Geometry: final body of the model. Coordinates: model frame, mm. A direction names the side the tool comes from. Round coordinates to 2 decimals unless told otherwise and drop trailing zeros. Loops run counter-clockwise (first coordinate to the right, second up) from the corner with the lowest first, then second, coordinate; pieces in that order, holes last. Notation, with made-up numbers: M -36.5,7 L -15.5,7 A13 cw -15.5,11 Z; hole C -12,84 d8. An arc over 180 degrees is marked long. Answer as a JSON object with one key per item and string values.
```python
from build123d import *

# Parameters (mm, degrees)
SKETCH1_R           = 2.5
BOSS_EXTRUDE1_DEPTH = 3.5
SKETCH2_R           = 1.5
CUT_EXTRUDE1_DEPTH  = 77.148499601
FILLET1_R           = 10
SKETCH5_R           = 15.25
SKETCH5_R_2         = 3
CUT_EXTRUDE4_DEPTH  = 77.148499601


with BuildPart() as part:
    # Sketch1 → Boss-Extrude1 (new body)
    with BuildSketch(Plane.XY):
        with BuildLine():
            Line((0, -19), (30, -19))
            Line((30, -19), (64.201367261, 15.201367261))
            Line((64.201367261, 15.201367261), (58.615223689, 20.787510832))
            Line((58.615223689, 20.787510832), (31.745166004, -6.082546853))
            Line((31.745166004, -6.082546853), (17.320187668, 8.342431483))
            Line((17.320187668, 8.342431483), (44.190245353, 35.212489168))
            Line((44.190245353, 35.212489168), (38.604101782, 40.798632739))
            Line((38.604101782, 40.798632739), (16.805469042, 19))
            Line((16.805469042, 19), (0, 19))
            ThreePointArc((0, 19), (-19, 0), (0, -19))
        make_face()
        Circle(SKETCH1_R, mode=Mode.SUBTRACT)
    extrude(amount=BOSS_EXTRUDE1_DEPTH)

    # Sketch2 → Cut-Extrude1 (cut, through all)
    with BuildSketch(Plane.XY.offset(3.5)):
        with Locations((38.878105659, 35.574881393)):
            Circle(SKETCH2_R)
        with Locations((58.977615915, 15.475371138)):
            Circle(SKETCH2_R)
    extrude(amount=-CUT_EXTRUDE1_DEPTH, mode=Mode.SUBTRACT)

    # Fillet1
    fillet1_edges = [part.edges().sort_by_distance(p)[0] for p in [
        (30, -19, 1.75),
        (16.805469042, 19, 1.75),
    ]]
    fillet(fillet1_edges, radius=FILLET1_R)

    # Sketch5 → Cut-Extrude4 (cut, through all)
    with BuildSketch(Plane.XY.offset(3.5)):
        Circle(SKETCH5_R)
        with Locations((38.878105659, 35.574881393)):
            Circle(SKETCH5_R_2)
        with Locations((58.977615915, 15.475371138)):
            Circle(SKETCH5_R_2)
    extrude(amount=-CUT_EXTRUDE4_DEPTH, mode=Mode.SUBTRACT)


solid = part.part
```
1) Line query: probe 1 along X at (y, z) = (-2.5, 2.85); probe 2 along X at (y, z) = (1.5, 1.55); probe 3 along X at (y, z) = (-7, 0.8). Output: solid intervals per line, ascending.
Geometry results:
{"probe 1": "-18.83 to -15.04, 15.04 to 28.16, 35.33 to 46.5", "probe 2": "-18.94 to -15.18, 15.18 to 24.16, 39.33 to 50.5", "probe 3": "-17.66 to -13.55, 13.55 to 42"}
2) Pull-direction query (X, two-part tool) for faces 1 (the face through (22, 2, 0)), 2 (the face through (29.301, 31.496, 1.726)), 3 (the face through (29.63, -18.26, 1.77)), 4 (the face through (-12.1, -9.28, 1.77)); classes: +X half, -X half, draft (parallel to the pull), parting line (faces both ways), or undercut.
Geometry results:
{"face 1": "draft", "face 2": "-X half", "face 3": "+X half", "face 4": "undercut"}
3) Cut plane A-A on x = 8.5. Return the cut outline in (y, z).
Geometry results:
{"outline": "M -19,0 L -12.66,0 L -12.66,3.5 L -19,3.5 Z; M 12.66,0 L 19,0 L 19,3.5 L 12.66,3.5 Z"}
4) Cut plane C-C on z = 1.2. Return the cut outline in (x, y), and give its area (3 significant figures).
Geometry results:
{"outline": "M 0,-19 L 25.86,-19 A10 ccw 32.93,-16.07 L 64.2,15.2 L 58.62,20.79 L 31.75,-6.08 L 17.32,8.34 L 44.19,35.21 L 38.6,40.8 L 19.73,21.93 A10 cw 12.66,19 L 0,19 A19 ccw Z; hole C 0,0 d30.5; hole C 38.88,35.57 d6; hole C 58.98,15.48 d6", "area": "1,330 mm2"}
5) Cut plane D-D on x = 51. Return the cut outline in (y, z).
Geometry results:
{"outline": "M 2,0 L 13.17,0 L 13.17,3.5 L 2,3.5 Z"}
6) First-contact query: pin 1 (7 mm diameter, centred on x = 58.98, y = 15.48, fed in from +Z); pin 2 (2 mm diameter, centred on x = 46, z = 2, fed in from -Y); pin 3 (1.8 mm diameter, centred on x = 5.5, z = 2.5, fed in from +Y); pin 4 (1.5 mm diameter, centred on x = 29, z = 2.5, fed in from -Y). Flat tips, straight axial feed; report the tip coordinate or a pass-through.
Geometry results:
{"pin 1": "z = 3.5", "pin 2": "y = -4", "pin 3": "y = 19", "pin 4": "y = -18.71"}
7) Cut plane B-B on y = 0. Return the cut outline in (x, z).
Geometry results:
{"outline": "M -19,0 L -15.25,0 L -15.25,3.5 L -19,3.5 Z; M 15.25,0 L 25.66,0 L 25.66,3.5 L 15.25,3.5 Z; M 37.83,0 L 49,0 L 49,3.5 L 37.83,3.5 Z"}
8) Set-up query: faces 5 (the face through (24.63, 1.03, 1.73)), 6 (the face through (6, 19, 2)), 7 (the face through (13, -19, 2)). Return all of +Z, -Z, +X, -X, +Y, -Y with unobstructed straight access to the full face (end or side cutting, diameter ignored); none if empty.
Geometry results:
{"face 5": "+Z, -Z", "face 6": "+Z, -Z, -X, +Y", "face 7": "+Z, -Z, +X, -X, -Y"}
